The listing builds one solid part. Answer for the finished solid, in the listing's coordinates (mm). A direction names the side the tool comes from. Round coordinates to 2 decimals unless told otherwise and drop trailing zeros. Write each loop counter-clockwise with the first axis right and the second up, starting at its lowest first coordinate (ties: lowest second). Pieces come first, ordered by that corner, then holes. Notation, with made-up numbers: M 53.25,-23 L 106.25,-23 A35 ccw 106.25,13 Z; hole C 26.5,41.25 d7. An arc over 180 degrees is marked long. Write each question's results on one line, items separated by ' | '.
from build123d import *

# Parameters (mm, degrees)
SKETCH1_R           = 2
SKETCH1_R_2         = 1
BOSS_EXTRUDE1_DEPTH = 7
SKETCH1_5_R         = 2
SKETCH1_5_R_2       = 1
CUT_EXTRUDE2_DEPTH  = 5
SKETCH1_6_R         = 3
SKETCH1_6_R_2       = 2
SKETCH1_6_R_3       = 1
BOSS_EXTRUDE3_DEPTH = 1
FILLET2_R           = 0.5
FILLET3_R           = 0.25
FILLET4_R           = 0.25
FILLET5_R           = 0.25


with BuildPart() as part:
    # Sketch1 → Boss-Extrude1 (new body)
    # profile 1 of 2: a face of its own
    with BuildSketch(Plane(origin=(0, 0, 0), x_dir=(1, 0, 0), z_dir=(0, 1, 0))):
        with Locations(Location((0, 0, 0), (0, 0, 270))):
            Circle(SKETCH1_R)
        Circle(SKETCH1_R_2, mode=Mode.SUBTRACT)
    # profile 2 of 2: a face of its own
    with BuildSketch(Plane(origin=(0, 0, 0), x_dir=(1, 0, 0), z_dir=(0, 1, 0))):
        Circle(SKETCH1_R_2)
    extrude(amount=BOSS_EXTRUDE1_DEPTH)

    # Sketch1_5 → Cut-Extrude2 (cut)
    with BuildSketch(Plane(origin=(0, 0, 0), x_dir=(1, 0, 0), z_dir=(0, 1, 0))):
        with Locations(Location((0, 0, 0), (0, 0, 270))):
            Circle(SKETCH1_5_R)
        with Locations(Location((0, 0, 0), (0, 0, 270))):
            Circle(SKETCH1_5_R_2, mode=Mode.SUBTRACT)
    extrude(amount=CUT_EXTRUDE2_DEPTH, mode=Mode.SUBTRACT)

    # Sketch1_6 → Boss-Extrude3 (add)
    # profile 1 of 2: a face of its own
    with BuildSketch(Plane(origin=(0, 0, 0), x_dir=(1, 0, 0), z_dir=(0, 1, 0))):
        with Locations(Location((0, 0, 0), (0, 0, 270))):
            Circle(SKETCH1_6_R)
        with Locations(Location((0, 0, 0), (0, 0, 270))):
            Circle(SKETCH1_6_R_2, mode=Mode.SUBTRACT)
    # profile 2 of 2: a face of its own
    with BuildSketch(Plane(origin=(0, 0, 0), x_dir=(1, 0, 0), z_dir=(0, 1, 0))):
        with Locations(Location((0, 0, 0), (0, 0, 270))):
            Circle(SKETCH1_6_R_2)
        with Locations(Location((0, 0, 0), (0, 0, 270))):
            Circle(SKETCH1_6_R_3, mode=Mode.SUBTRACT)
    extrude(amount=BOSS_EXTRUDE3_DEPTH)

    # Fillet2
    fillet2_edges = [part.edges().sort_by_distance(p)[0] for p in [
        (0, 7, -2),
    ]]
    fillet(fillet2_edges, radius=FILLET2_R)

    # Fillet3
    fillet3_edges = [part.edges().sort_by_distance(p)[0] for p in [
        (0, 1, -3),
    ]]
    fillet(fillet3_edges, radius=FILLET3_R)

    # Fillet4
    fillet4_edges = [part.edges().sort_by_distance(p)[0] for p in [
        (0, 5, -1),
        (0, 5, -2),
    ]]
    fillet(fillet4_edges, radius=FILLET4_R)

    # Fillet5
    fillet5_edges = [part.edges().sort_by_distance(p)[0] for p in [
        (0, 1, -1),
    ]]
    fillet(fillet5_edges, radius=FILLET5_R)


solid = part.part
1) A tool of negligible diameter and unlimited length cuts with its end or side. For faces 4 (the face through (-1, 1, 1)), 5 (the face through (0, 7, 0)), from which of +Z, -Z, +X, -X, +Y, -Y can it reach the whole face along a straight path? Write none if from no direction.
Return value:
face 4: none | face 5: +Z, -Z, +X, -X, +Y
2) Section B-B (x = 0) is taken. Determine the outline of the cut face in (y, z), then the cut area to 3 significant figures.
Return value:
outline: M 0,-3 L 0.75,-3 A0.25 ccw 1,-2.75 L 1,-1.25 A0.25 cw 1.25,-1 L 4.75,-1 A0.25 cw 5,-1.25 L 5,-1.75 A0.25 ccw 5.25,-2 L 6.5,-2 A0.5 ccw 7,-1.5 L 7,1.5 A0.5 ccw 6.5,2 L 5.25,2 A0.25 ccw 5,1.75 L 5,1.25 A0.25 cw 4.75,1 L 1.25,1 A0.25 cw 1,1.25 L 1,2.75 A0.25 ccw 0.75,3 L 0,3 Z | area: 21.9 mm²
3) Section C-C (y = 2.25) is taken. Determine the outline of the cut face in (x, z), then the cut area to 3 significant figures.
Return value:
outline: C 0,0 d2 | area: 3.14 mm²
4) Section A-A (z = 0) is taken. Determine the outline of the cut face in (x, y).
Return value:
outline: M -3,0 L 3,0 L 3,0.75 A0.25 ccw 2.75,1 L 1.25,1 A0.25 cw 1,1.25 L 1,4.75 A0.25 cw 1.25,5 L 1.75,5 A0.25 ccw 2,5.25 L 2,6.5 A0.5 ccw 1.5,7 L -1.5,7 A0.5 ccw -2,6.5 L -2,5.25 A0.25 ccw -1.75,5 L -1.25,5 A0.25 cw -1,4.75 L -1,1.25 A0.25 cw -1.25,1 L -2.75,1 A0.25 ccw -3,0.75 Z
5) The mould has two halves that part along Y. Classify faces 1 (the face through (-2, 6, 0)), 2 (the face through (0, 0, 0)), 3 (the face through (-1, 5, 1)): +Y half, -Y half, draft (parallel to the pull), parting line (faces both ways), or undercut.
Return value:
face 1: draft | face 2: -Y half | face 3: undercut
6) Each of these flat-tipped pins is pushed along its axis until it touches: pin 1 (1.5 mm diameter, centred on x = -1, y = 4.5, fed in from +Z); pin 2 (2 mm diameter, centred on x = 2, y = 1.5, fed in from +Z); pin 3 (2 mm diameter, centred on y = 1.5, z = -1.5, fed in from +X). Where does it stop, or does it pass through?
Return value:
pin 1: z = 1.88 | pin 2: z = 2.71 | pin 3: x = 2.89
7) Find the intervals of material crossed by line 1 (Y direction, x = 0.75, z = 2); line 2 (Y direction, x = 0.5, z = -1.75); line 3 (Y direction, x = -0.75, z = 1.5), in increasing order.
Return value:
line 1: 0 to 1 | line 2: 0 to 1, 5.01 to 6.88 | line 3: 0 to 1, 5 to 6.97
